from build123d import *

# Parameters (mm, degrees)
SZKIC1_W                    = 394
SZKIC1_H                    = 77
DODANIE_WYCI_GNI_CIE1_DEPTH = 5
WYTNIJ_WYCI_GNI_CIE1_DEPTH  = 10


with BuildPart() as part:
    # Szkic1 → Dodanie-wyciągnięcie1 (new body)
    with BuildSketch(Plane.XY):
        with Locations((-82.604690639, -71.272983114)):
            Rectangle(SZKIC1_W, SZKIC1_H)
    extrude(amount=DODANIE_WYCI_GNI_CIE1_DEPTH)

    # Szkic2 → Wytnij-wyciągnięcie1 (cut)
    with BuildSketch(Plane.XY.offset(5)):
        with BuildLine():
            Line((-255.604690639, -39.772983114), (90.395309361, -39.772983114))
            ThreePointArc((90.395309361, -39.772983114), (97.466377173, -42.701915303), (100.395309361, -49.772983114))
            Line((100.395309361, -49.772983114), (100.395309361, -92.772983114))
            ThreePointArc((100.395309361, -92.772983114), (97.466377173, -99.844050926), (90.395309361, -102.772983114))
            Line((90.395309361, -102.772983114), (-255.604690639, -102.772983114))
            ThreePointArc((-255.604690639, -102.772983114), (-262.675758451, -99.844050926), (-265.604690639, -92.772983114))
            Line((-265.604690639, -92.772983114), (-265.604690639, -49.772983114))
            ThreePointArc((-265.604690639, -49.772983114), (-262.675758451, -42.701915303), (-255.604690639, -39.772983114))
        make_face()
    extrude(amount=-WYTNIJ_WYCI_GNI_CIE1_DEPTH, mode=Mode.SUBTRACT)


solid = part.part
Source: CAD feature listing. Evaluate the final solid. Frame: model axes, mm. A direction names the side the tool comes from. Give positions to 0.01 mm unless a question says otherwise; leave off trailing zeros. Write each loop counter-clockwise with the first axis right and the second up, starting at its lowest first coordinate (ties: lowest second). Pieces come first, ordered by that corner, then holes. Notation, with made-up numbers: (61, 24) -> (115, 24) arc R9 ccw to (115, 33) -> close; hole circle Ø11 at (84, 84). An arc over 180 degrees is marked (long way). Return JSON: item names as keys, results as strings. Group by question number.
1. Section B-B, the plane y = -76. Output: boundary loops of the cut face in (x, z).
2. Material intervals for line 1 (Y direction, x = 12.5, z = 1.2); line 2 (X direction, y = -75.5, z = 2.6); line 3 (Y direction, x = 91.5, z = 1.15), sorted ascending. Write a range as from..to.
3. Mould query, pull axis X, two halves, no side actions, for faces 3 (the face through (-98, -37, 5)), 4 (the face through (-262.6, -99.92, 2.54)). Classes: +X half, -X half, draft (parallel to the pull), parting line (faces both ways), or undercut.
4. Section C-C, the plane z = 1.6. Output: boundary loops of the cut face in (x, y).
5. Access query for faces 1 (the face through (97.54, -99.77, 2.54)), 2 (the face through (-98, -37, 0)). Directions: +Z, -Z, +X, -X, +Y, -Y. A direction counts if a zero-diameter tool reaches every point of the face in a straight line with its end or side. Return the directions, or none.
6. Section A-A, the plane x = -98. Output: boundary loops of the cut face in (y, z).
Determined:
{
 "1": {"outline": "(-279.6, 0) -> (-265.6, 0) -> (-265.6, 5) -> (-279.6, 5) -> close; (100.4, 0) -> (114.4, 0) -> (114.4, 5) -> (100.4, 5) -> close"},
 "2": {"line 1": "y = -109.77..-102.77, -39.77..-32.77", "line 2": "x = -279.6..-265.6, 100.4..114.4", "line 3": "y = -109.77..-102.71, -39.83..-32.77"},
 "3": {"face 3": "draft", "face 4": "undercut"},
 "4": {"outline": "(-279.6, -109.77) -> (114.4, -109.77) -> (114.4, -32.77) -> (-279.6, -32.77) -> close; hole (-265.6, -92.77) arc R10 ccw to (-255.6, -102.77) -> (90.4, -102.77) arc R10 ccw to (100.4, -92.77) -> (100.4, -49.77) arc R10 ccw to (90.4, -39.77) -> (-255.6, -39.77) arc R10 ccw to (-265.6, -49.77) -> close"},
 "5": {"face 1": "+Z, -Z", "face 2": "-Z, +X, -X, +Y, -Y"},
 "6": {"outline": "(-109.77, 0) -> (-102.77, 0) -> (-102.77, 5) -> (-109.77, 5) -> close; (-39.77, 0) -> (-32.77, 0) -> (-32.77, 5) -> (-39.77, 5) -> close"}
}
